For this review, use the dimensioned drawing (mm, ordinates from the lowest corner) and the shaded views. A direction names the side the tool comes from. Give positions to 0.01 mm unless a question says otherwise; leave off trailing zeros. Write each loop counter-clockwise with the first axis right and the second up, starting at its lowest first coordinate (ties: lowest second). Pieces come first, ordered by that corner, then holes.
1) We need section A-A on y = 13. Give the boundary of the cut face in (x, z).
2) Wall thickness on line 1 along X through (y, z) = (4.25, 3.35); line 2 along Z through (x, y) = (1.5, 22.75); line 3 along Z through (x, y) = (7.25, 6.75): over which ranges is each line inside the solid? List them lowest first.
3) We need section B-B on z = 4.2. Give the boundary of the cut face in (x, y).
4) For P1, Ø3.5, axis at x = 6.5, y = 10, coming from the +Z side; P2, Ø0.5, axis at x = 2, z = 3.5, coming from the +Y side (1 decimal); P3, Ø2.5, axis at x = 1, y = 12, coming from the -Z side; P4, Ø0.5, axis at x = 2, z = 4, coming from the -Y side (1 decimal), all flat-tipped, find the tip position at first contact; note any pin that passes through.
5) Draft analysis for pull direction X (two halves, no side actions). For the marked faces 1, 2, 3 and 4, state which applies: pulls with the +X half, pulls with the -X half, needs draft (parallel to the pull), parting line crosses it, or undercut.
6) We need section C-C on x = 2.75. Give the boundary of the cut face in (y, z).
7) We need section D-D on z = 0.6. Give the boundary of the cut face in (x, y).
8) Machinability: for the marked faces 5, 6, 7, 8 and 9, which of the approach directions +Z, -Z, +X, -X, +Y, -Y give a long, thin tool a straight path to every point of the face, cutting with its end or side? Answer none if there is none.
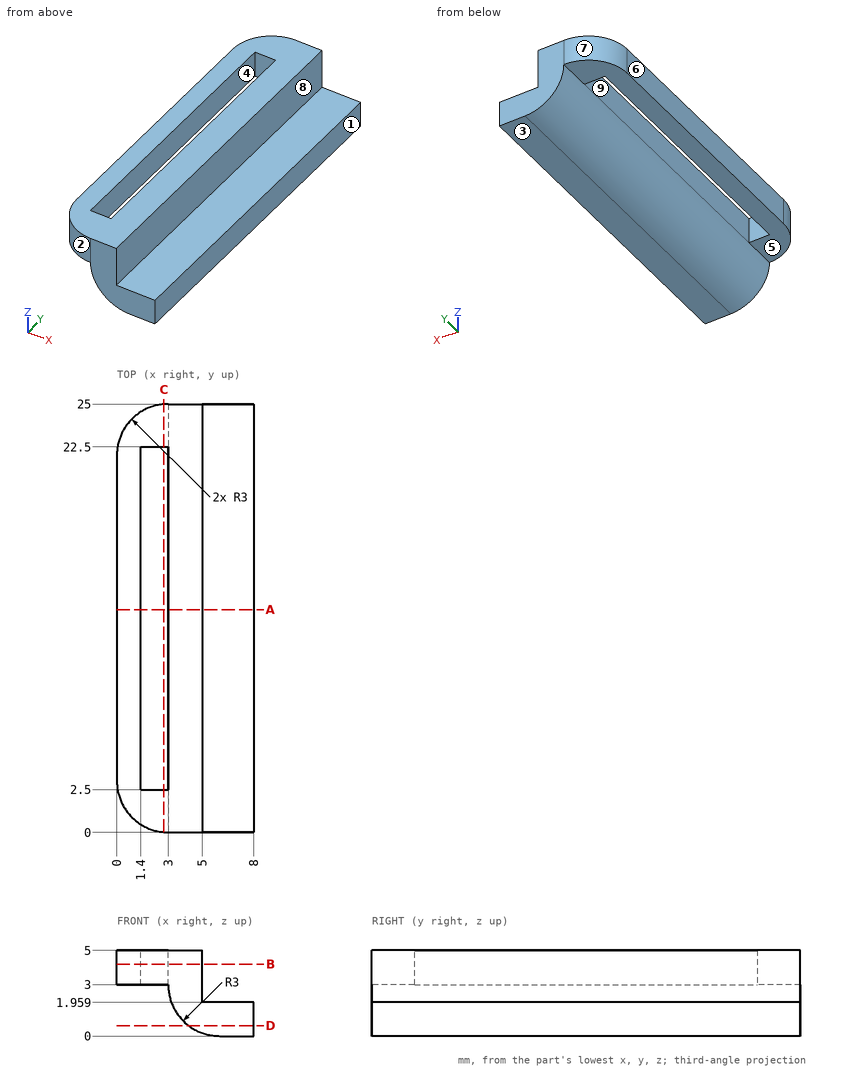
Results list:
1. outline: (0, 3) - (1.4, 3) - (1.4, 5) - (0, 5) - close; (3, 3) arc R3 ccw to (6, 0) - (8, 0) - (8, 1.96) - (5, 1.96) - (5, 5) - (3, 5) - close
2. line 1: x = 0 to 1.4, 3 to 5
2. line 2: z = 3 to 5
2. line 3: z = 0 to 1.96
3. outline: (0, 3) arc R3 ccw to (3, 0) - (5, 0) - (5, 25) - (3, 25) arc R3 ccw to (0, 22) - close; hole (1.4, 2.5) - (3, 2.5) - (3, 22.5) - (1.4, 22.5) - close
4. P1: stops at z = 5
4. P2: stops at y = 24.9
4. P3: stops at z = 3
4. P4: stops at y = 0.1
5. face 1: pulls with the +X half
5. face 2: pulls with the -X half
5. face 3: needs draft
5. face 4: undercut
6. outline: (0.01, 3) - (2.5, 3) - (2.5, 5) - (0.01, 5) - close; (22.5, 3) - (24.99, 3) - (24.99, 5) - (22.5, 5) - close
7. outline: (4.2, 0) - (8, 0) - (8, 25) - (4.2, 25) - close
8. face 5: -Z, -X, +Y, -Y
8. face 6: +Z, -Z, -X, +Y, -Y
8. face 7: +Z, -Z, -X, +Y
8. face 8: +Z, +X, +Y, -Y
8. face 9: +Z, -Z
